Here's how the part is built. I have some questions about the finished solid (model axes, mm). Face numbers are marked on the shaded views. A direction names the side the tool comes from. Coordinates: 2 decimals unless noted, no trailing zeros. Write each loop counter-clockwise with the first axis right and the second up, starting at its lowest first coordinate (ties: lowest second). Pieces come first, ordered by that corner, then holes. Notation, with made-up numbers: M -3,65.25 L 4,65.25 A25 ccw 4,78.25 Z; hole C 13,70 d4. An arc over 180 degrees is marked long. Use one line per item in the form item = value. Start each with the question number.
1. I want a section at C-C, the plane y = -8.25. List the corners of the cut face in (x, z) for me, plus the area to 3 significant figures.
2. I want a section at D-D, the plane z = 3.5. List the corners of the cut face in (x, y) for me, plus the area to 3 significant figures.
3. On a 3-axis mill with a long thin cutter (end or side, diameter ignored), from which of +Z, -Z, +X, -X, +Y, -Y can I reach the whole of each face in a straight line? I mean the marked faces 1 and 2. Say none if no direction works.
4. I want a section at A-A, the plane z = 6. List the corners of the cut face in (x, y) for me, plus the area to 3 significant figures.
5. Please list where these lines run through material, in increasing order: line 1 along X through (y, z) = (-5, 3.7); line 2 along Y through (x, z) = (2.5, 3.45); line 3 along Z through (x, y) = (7.5, -5.25). Write a range as [from, to].
6. Thinking about a two-plate mould opening in Z: for the marked faces 3, 4 and 5, which applies, released by +Z, released by -Z, zero draft, split by the parting line, or undercut?
7. I want a section at B-B, the plane x = 7.5. List the corners of the cut face in (y, z) for me.
8. I'm going to push flat-ended pins straight in: pin 1 Ø1 at (y, z) = (-5, 13.5) entering from +X; pin 2 Ø2 at (x, y) = (4, -2) entering from +Z; pin 3 Ø0.8 at (x, y) = (2.5, -5) entering from -Z. Where does each tip first touch, or does it pass through?
from build123d import *

# Parameters (mm, degrees)
F0_R     = 5
F1_DEPTH = 10
F2_R     = 1.25
F3_DEPTH = 5


with BuildPart() as f1:
    # F0 (on Front) → F1 (new body)
    with BuildSketch(Plane.XZ):
        with BuildLine():
            Line((0, 10), (0, 0))
            Line((0, 0), (15, 0))
            Line((15, 0), (15, 10))
            ThreePointArc((15, 10), (7.5, 17.5), (0, 10))
        make_face()
        with Locations((7.5, 10)):
            Circle(F0_R, mode=Mode.SUBTRACT)
    extrude(amount=F1_DEPTH)

    # F2 (on face) → F3 (cut)
    with BuildSketch(Plane(origin=(0, 0, 0), x_dir=(1, 0, 0), z_dir=(0, 0, -1))):
        with Locations((2.5, 5)):
            Circle(F2_R)
        with Locations((12.5, 5)):
            Circle(F2_R)
    extrude(amount=-F3_DEPTH, mode=Mode.SUBTRACT)


solid = f1.part
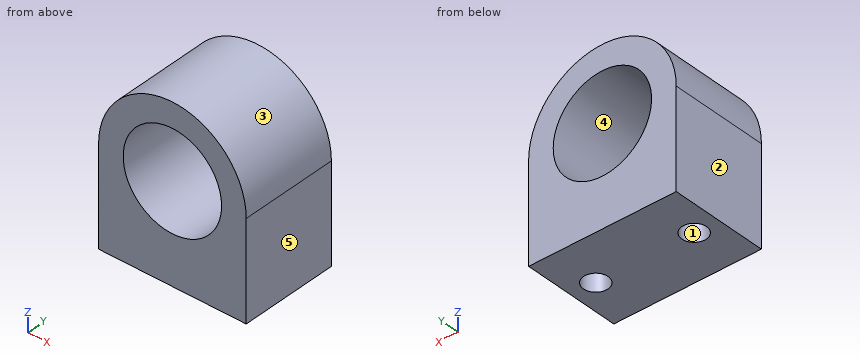
Answer list:
q1.outline = M 0,0 L 15,0 L 15,10 A7.5 ccw 0,10 Z; hole C 7.5,10 d10
q1.area = 160 mm²
q2.outline = M 0,-10 L 15,-10 L 15,0 L 0,0 Z; hole C 2.5,-5 d2.5; hole C 12.5,-5 d2.5
q2.area = 140 mm²
q3.face_1 = -Z
q3.face_2 = +Z, -Z, -X, +Y, -Y
q4.outline = M 0,-10 L 4.5,-10 L 4.5,0 L 0,0 Z; M 10.5,-10 L 15,-10 L 15,0 L 10.5,0 Z
q4.area = 90.0 mm²
q5.line_1 = [0, 1.25], [3.75, 11.25], [13.75, 15]
q5.line_2 = [-10, -6.25], [-3.75, 0]
q5.line_3 = [0, 5], [15, 17.5]
q6.face_3 = released by +Z
q6.face_4 = undercut
q6.face_5 = zero draft
q7.outline = M -10,0 L 0,0 L 0,5 L -10,5 Z; M -10,15 L 0,15 L 0,17.5 L -10,17.5 Z
q8.pin_1 = 14.37
q8.pin_2 = 17.07
q8.pin_3 = 5
